Autodesk Inventor part; units mm, degrees
ref_plane "YZ Plane" through (0, 0, 0) normal (1, 0, 0) x (0, 1, 0)
ref_plane "XZ Plane" through (0, 0, 0) normal (0, 1, 0) x (-1, 0, 0)
ref_plane "XY Plane" through (0, 0, 0) normal (0, 0, 1) x (1, 0, 0)
sketch "Sketch1" plane through (0, 0, 0) normal (1, 0, 0) x (0, 1, 0)
  line L0 (15, 15) -> (-15, 15)
  line L1 (-15, -15) -> (15, -15)
  line L2 (15, -15) -> (15, 15)
  line L3 (15, 15) -> (-15, -15) construction
  line L4 (-15, 15) -> (15, -15) construction
  line L5 (-15, -15) -> (-25, -15)
  line L6 (-25, -15) -> (-25, 15)
  line L7 (-25, 15) -> (-15, 15)
  point P0 (0, 0)
  dimension "d0" = 30
  dimension "d1" = 30
  dimension "d13" = 10
extrude "Extrusion1" add sketch "Sketch1" along normal blind 10
sketch "Sketch2" plane through (0, 0, 0) normal (-1, 0, 0) x (0, 0, 1)
  line L0 (-13, -13) -> (-13, 13)
  line L1 (13, 13) -> (13, -13)
  line L2 (13, 13) -> (-13, 13)
  line L3 (-13, -13) -> (-13, -23)
  line L4 (-13, -23) -> (13, -23)
  line L5 (13, -23) -> (13, -13)
  point P0 (0, 0)
  dimension "d14" = 10
extrude "Extrusion2" cut sketch "Sketch2" against normal blind 8
sketch "Sketch3" plane through (0, 15, 15) normal (0, 1, 0) x (1, 0, 0)
  circle A0 centre (4.4342, 15) radius 2.5
  point P0 (0, 15)
extrude "Extrusion3" add sketch "Sketch3" along normal blind 5
sketch "Sketch4" plane through (0, 13, -13) normal (0, -1, 0) x (1, 0, 0)
  circle A0 centre (4.4342, 23) radius 1.225
  circle A1 centre (4.4342, 3) radius 1.225
  point P0 (0, 13)
extrude "Extrusion4" cut sketch "Sketch4" against normal blind 2
fillet "Fillet4" radius 8 4 edges at (4, -23, 13) (4, -23, -13) (5, -25, -15) (5, -25, 15)
fillet "Fillet5" radius 4 4 edges at (10, -25, 0) (10, -22.6569, 12.6569) (10, -1, -15) (10, -22.6569, -12.6569)
sketch "Sketch5" plane through (8, 0, 0) normal (-1, 0, 0) x (0, 0, 1)
  arc A0 (12.525, -5.1293) -> (-12.525, -5.1293) centre (0, -5.1293) ccw
  circle A1 centre (0, -5.1293) radius 11.025
  arc A2 (5, -23) -> (13, -15) centre (5, -15) ccw
  line L0 (13, -5.1293) -> (13, -15)
  line L1 (5, -23) -> (-5, -23)
  arc A3 (-13, -15) -> (-5, -23) centre (-5, -15) ccw
  line L2 (-13, -15) -> (-13, -5.1293)
  line L3 (12.525, -5.1293) -> (13, -5.1293)
  line L4 (13, -5.1293) -> (13, -15)
  line L5 (-12.525, -5.1293) -> (-13, -5.1293)
  line L6 (-13, -15) -> (-13, -5.1293)
  point P0 (0, 0)
extrude "Extrusion5" add sketch "Sketch5" along normal blind 8
sketch "Sketch6" plane through (8, -5.1293, 0) normal (-1, 0, 0) x (0, 0, 1)
  circle A0 centre (0, 0) radius 11.025
  point P0 (0, 5.1293)
extrude "Extrusion6" add sketch "Sketch6" along normal blind 4.5
sketch "Sketch7" plane through (10, 0, 0) normal (1, 0, 0) x (0, 0, -1)
  circle A0 centre (0, -5.1293) radius 1.525
  point P0 (0, 0)
extrude "Extrusion7" cut sketch "Sketch7" against normal blind 8
sketch "Sketch8" plane through (10, 0, 0) normal (1, 0, 0) x (0, 0, -1)
  circle A0 centre (0, -5.1293) radius 1.525
  circle A1 centre (0, -5.1293) radius 3
  point P0 (0, 0)
  dimension "d29" = 6
extrude "Extrusion8" cut sketch "Sketch8" against normal blind 5
sketch "Sketch9" plane through (10, 0, 0) normal (1, 0, 0) x (0, 0, -1)
  circle A0 centre (0, -5.1293) radius 11.025
  line L0 (0, -5.1293) -> (0, -13.0693)
  line L1 (0, -5.1293) -> (0, 2.8107)
  circle A1 centre (0, -5.1293) radius 1.525
  line L2 (0, -5.1293) -> (7.94, -5.1293)
  line L3 (0, -5.1293) -> (-7.94, -5.1293)
  circle A2 centre (7.94, -5.1293) radius 1.59
  circle A3 centre (0, -13.0693) radius 1.59
  circle A4 centre (-7.94, -5.1293) radius 1.59
  circle A5 centre (0, 2.8107) radius 1.59
  point P0 (0, 0)
  dimension "d32" = 7.94
  dimension "d33" = 7.94
  dimension "d34" = 7.94
  dimension "d35" = 7.94
  dimension "d36" = 3.18
  dimension "d37" = 3.18
  dimension "d38" = 3.18
  dimension "d39" = 3.18
extrude "Extrusion9" cut sketch "Sketch9" against normal blind 8 contours A3 | A4 | A5 | A2
sketch "Sketch10" plane through (10, 0, 0) normal (1, 0, 0) x (0, 0, -1)
  circle A0 centre (0, 2.8107) radius 1.59
  circle A1 centre (7.94, -5.1293) radius 1.59
  circle A2 centre (0, -13.0693) radius 1.59
  circle A3 centre (-7.94, -5.1293) radius 1.59
  circle A4 centre (0, 2.8107) radius 2.5
  circle A5 centre (7.94, -5.1293) radius 2.5
  circle A6 centre (0, -13.0693) radius 2.5
  circle A7 centre (-7.94, -5.1293) radius 2.5
  point P0 (0, 0)
  dimension "d42" = 5
  dimension "d43" = 5
  dimension "d44" = 5
  dimension "d45" = 5
extrude "Extrusion10" cut sketch "Sketch10" against normal blind 5
properties part number "TapaPieEfector"
Input: part model. Units: mm. Frame: model coordinates. A direction names the side the tool comes from. Give positions to 0.01 mm unless a question says otherwise; leave off trailing zeros. Write each loop counter-clockwise with the first axis right and the second up, starting at its lowest first coordinate (ties: lowest second). Pieces come first, ordered by that corner, then holes. Notation, with made-up numbers: M 85,78.5 L 116,78.5 A26 ccw 116,115.5 Z; hole C 25,7.25 d8. An arc over 180 degrees is marked long. Write item = value, one per line. Start each with the question number.
1) First-contact query: pin 1 Ø9 at (y, z) = (7.5, -4.5) entering from -X; pin 2 Ø1.5 at (y, z) = (-4.5, 7) entering from +X; pin 3 Ø2 at (x, z) = (1.5, -4.5) entering from +Y; pin 4 Ø3 at (y, z) = (-5.13, -7.94) entering from +X (3 decimals). Flat tips, straight axial feed; report the tip coordinate or a pass-through.
2) Material intervals for line 1 along Y through (x, z) = (4.75, 7.94); line 2 along Y through (x, z) = (2.7, 0); line 3 along Z through (x, y) = (4.75, 8), sorted ascending. Write a range as [from, to].
3) Reachability of faces 5 (the cylindrical face through (7.535, -4.378, 5.555)), 6 (the flat face through (0, 0, -10)) from +Z, -Z, +X, -X, +Y, -Y: full face, straight path, thin tool, end or side. Return the list, or none.
4) Cut plane A-A on x = 1. Return the cut outline in (y, z) (3 decimals).
5) Cut plane B-B on z = 0. Count the separate pieces of the cut face and the enclosed holes in it, then the cut area to 3 significant figures.
6) Draft query along X for faces 1 (the flat face through (5, -6.4, -1.3)), 2 (the cylindrical face through (6.744, 17.465, -0.958)), 3 (the cylindrical face through (5.566, 13.986, -10.469)), 4 (the cylindrical face through (4.26, -5.74, -9.41)). Return one class per face: +X half, -X half, draft (parallel to the pull), parting line (faces both ways), or undercut.
Solved:
q1.pin_1 = 0
q1.pin_2 = 5
q1.pin_3 = 15
q1.pin_4 = through
q2.line_1 = [-24.94, -6.72], [-3.54, 4.56], [13, 15]
q2.line_2 = [-25, -16.15], [5.9, 7.4], [13, 20]
q2.line_3 = [-15, -13], [13, 15]
q3.face_5 = +X
q3.face_6 = +Z, -Z, -X, +Y, -Y
q4.outline = M -25,-7 A8 ccw -17,-15 L 15,-15 L 15,15 L -17,15 A8 ccw -25,7 Z; hole C -5.129,0 d22.05; hole M -5.129,-13 L 13,-13 L 13,13 L -5.129,13 L -5.129,12.525 A12.525 cw -5.129,-12.525 Z
q5.separate_pieces = 4
q5.enclosed_holes = 0
q5.area = 205 mm2
q6.face_1 = +X half
q6.face_2 = parting line
q6.face_3 = undercut
q6.face_4 = draft
